Build history of the part. All positions in model axes, mm. Face numbers are marked on the shaded views. A direction names the side the tool comes from. Give positions to 0.01 mm unless a question says otherwise; leave off trailing zeros. Order: outer loops, then holes, each group sorted by start corner. A loop starts at its lowest first (then second) coordinate and runs counter-clockwise, first axis right, second up. Notation, with made-up numbers: (40, -14.5) - (85, -14.5) arc R16 cw to (85, 10.5) - close; hole circle Ø4 at (27, -13). An arc over 180 degrees is marked (long way). Answer in a Markdown table with one row per item.
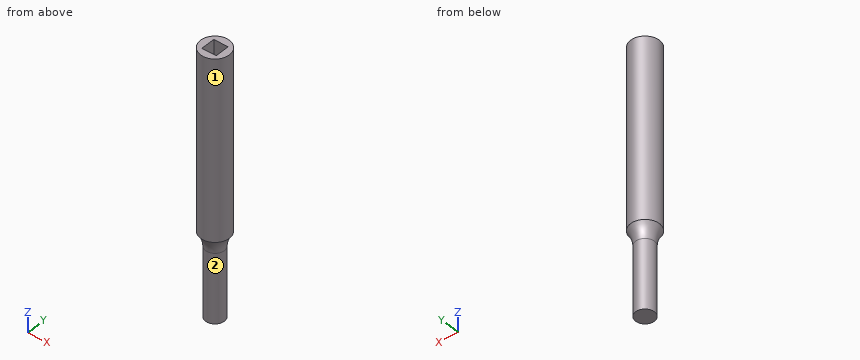
```python
from build123d import *

# Parameters (mm, degrees)
SKETCH5_R           = 3.9
BOSS_EXTRUDE4_DEPTH = 35
SKETCH6_R           = 6
BOSS_EXTRUDE5_DEPTH = 75
FILLET1_R           = 10
SKETCH7_W           = 6
SKETCH7_H           = 6
CUT_EXTRUDE1_DEPTH  = 20


with BuildPart() as part:
    # Sketch5 → Boss-Extrude4 (new body)
    with BuildSketch(Plane.XY):
        Circle(SKETCH5_R)
    extrude(amount=BOSS_EXTRUDE4_DEPTH)

    # Sketch6 → Boss-Extrude5 (add)
    with BuildSketch(Plane.XY.offset(35)):
        Circle(SKETCH6_R)
    extrude(amount=BOSS_EXTRUDE5_DEPTH)

    # Fillet1
    # the kernel refuses this fillet: 10 mm, written as the material it adds along each edge
    with BuildSketch(Plane(origin=(0, 0, 35), x_dir=(1, 0, 0), z_dir=(0, -1, 0))) as fillet1_piece_1:
        with BuildLine():
            CenterArc((13.9, -6.131068422), FILLET1_R, 142.185511494, 37.814488506)
            Line((3.9, -6.131068422), (3.7, -6.131068422))
            Line((3.7, -6.131068422), (3.7, 0))
            Line((3.7, 0), (3.9, 0.2))
            ThreePointArc((3.9, 0.2), (4.95, 0.2), (5.842, 0.122621368))
            Line((5.842, 0.122621368), (6, 0))
        make_face()
    revolve(axis=Axis((0, 0, 35), (0, 0, 1)))

    # Sketch7 → Cut-Extrude1 (cut)
    with BuildSketch(Plane.XY.offset(110)):
        Rectangle(SKETCH7_W, SKETCH7_H)
    extrude(amount=-CUT_EXTRUDE1_DEPTH, mode=Mode.SUBTRACT)


solid = part.part
```
1. Cut at D-D on z = 78. Write the cut outline in (x, y).
Check result:
| item | result |
|---|---|
| outline | circle Ø12 at (0, 0) |
2. Probe line 1 (Y direction, x = -0.5, z = 97.5); line 2 (Z direction, x = 2, y = 2); line 3 (X direction, y = 0.25, z = 70). List the from-to ranges inside material, lowest first.
Check result:
| item | result |
|---|---|
| line 1 | y = -5.98 to -3, 3 to 5.98 |
| line 2 | z = 0 to 90 |
| line 3 | x = -5.99 to 5.99 |
3. Cut at A-A on y = 0. Write the cut outline in (x, z).
Check result:
| item | result |
|---|---|
| outline | (-6, 35) arc R10 cw to (-3.9, 28.87) - (-3.9, 0) - (3.9, 0) - (3.9, 28.87) arc R10 cw to (6, 35) - (6, 110) - (3, 110) - (3, 90) - (-3, 90) - (-3, 110) - (-6, 110) - close |
4. Drop flat-ended pins along their axis: P1, Ø6, axis at y = 5, z = 29, coming from the -X side; P2, Ø4, axis at x = -4, z = 27.5, coming from the -Y side; P3, Ø1.5, axis at x = 0.5, y = 0, coming from the +Z side. Give the stop position or say it passes through.
Check result:
| item | result |
|---|---|
| P1 | stops at x = -3.35 |
| P2 | stops at y = -3.35 |
| P3 | stops at z = 90 |
5. Cut at C-C on z = 25. Write the cut outline in (x, y).
Check result:
| item | result |
|---|---|
| outline | circle Ø7.8 at (0, 0) |
6. Which spindle directions (+Z, -Z, +X, -X, +Y, -Y) get a long thin tool onto all of the face, cutting with end or side? Do the marked faces 1 and 2. Say none if no direction does.
Check result:
| item | result |
|---|---|
| face 1 | +Z, -Z |
| face 2 | -Z |
